Check sheet for the drawn part. Datum: minimum x, y, z corner. Units: mm. A direction names the side the tool comes from. Coordinates: 2 decimals unless noted, no trailing zeros. Write each loop counter-clockwise with the first axis right and the second up, starting at its lowest first coordinate (ties: lowest second). Pieces come first, ordered by that corner, then holes. Notation, with made-up numbers: M 67.5,-4.75 L 121.5,-4.75 A32 ccw 121.5,25.25 Z; hole C 45.5,53 d1. An arc over 180 degrees is marked long. Answer as CSV lines item,"result".
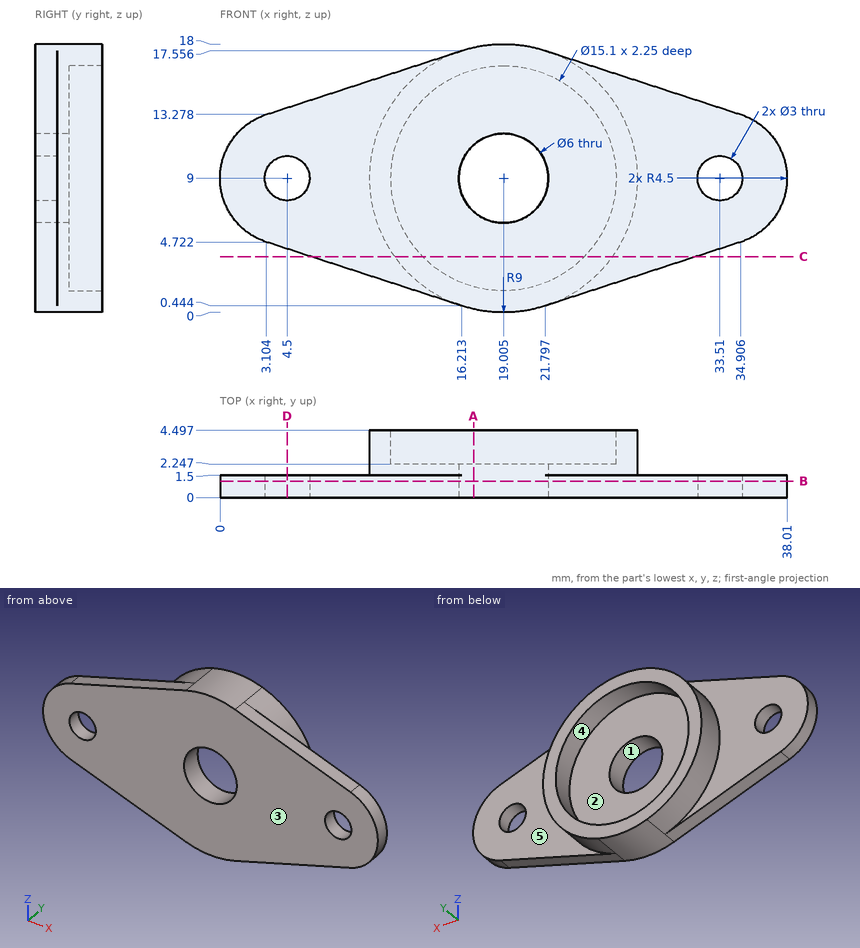
1) Section check B-B, the plane y = 1.1. Record the boundary of the cut face in (x, z) (1 decimal), plus the area to 3 significant figures.
Answer key:
outline,"M 3.1,4.7 L 16.2,0.4 A9 ccw 21.8,0.4 L 34.9,4.7 A4.5 ccw 34.9,13.3 L 21.8,17.6 A9 ccw 16.2,17.6 L 3.1,13.3 A4.5 ccw Z; hole C 4.5,9 d3; hole C 19,9 d6; hole C 33.5,9 d3"
area,"432 mm2"
2) Section check A-A, the plane x = 17. Record the boundary of the cut face in (y, z).
Answer key:
outline,"M 0,0.23 L 4.5,0.23 L 4.5,1.72 L 2.25,1.72 L 2.25,6.77 L 0,6.77 Z; M 0,11.23 L 2.25,11.23 L 2.25,16.28 L 4.5,16.28 L 4.5,17.77 L 0,17.77 Z"
3) Thickness scan on line 1 along Y through (x, z) = (35.5, 9.75); line 2 along Z through (x, y) = (5.5, 1.4); line 3 along Y through (x, z) = (22.5, 11.5). Record the ranges inside material, lowest first.
Answer key:
line 1,"y = 0 to 1.5"
line 2,"z = 3.94 to 7.88, 10.12 to 14.06"
line 3,"y = 0 to 2.25"
4) Tool access check on the marked faces 4 and 5. Record the directions out of +Z, -Z, +X, -X, +Y, -Y that give a thin tool (end or side, any length) a straight path to the whole face; none if there is none.
Answer key:
face 4,"+Y"
face 5,"+X, +Y"
5) Depth check by flat-ended pin: P1, Ø4.5, axis at x = 19.5, z = 11, coming from the +Y side; P2, Ø2.5, axis at x = 4.5, z = 9, coming from the -Y side; P3, Ø5, axis at x = 33.51, z = 9, coming from the +Y side. Enter the tip coordinate at first touch or a pass-through.
Answer key:
P1,"stops at y = 2.25"
P2,"passes through"
P3,"stops at y = 1.5"
6) Section check C-C, the plane z = 3.75. Record the boundary of the cut face in (x, y) (1 decimal).
Answer key:
outline,"M 6.1,0 L 31.9,0 L 31.9,1.5 L 26.3,1.5 L 26.3,4.5 L 24.4,4.5 L 24.4,2.2 L 13.6,2.2 L 13.6,4.5 L 11.7,4.5 L 11.7,1.5 L 6.1,1.5 Z"
7) Mould release check, pull along Z, two halves, no side actions. Record for the marked faces 1, 2 and 3: pulls with the +Z half, pulls with the -Z half, needs draft (parallel to the pull), parting line crosses it, or undercut.
Answer key:
face 1,"undercut"
face 2,"undercut"
face 3,"needs draft"
8) Section check D-D, the plane x = 4.5. Record the boundary of the cut face in (y, z).
Answer key:
outline,"M 0,4.27 L 1.5,4.27 L 1.5,7.5 L 0,7.5 Z; M 0,10.5 L 1.5,10.5 L 1.5,13.73 L 0,13.73 Z"
